```python
from build123d import *

# Parameters (mm, degrees)
SALIENTE_EXTRUIR1_DEPTH = 8.98
CROQUIS2_R              = 7
SALIENTE_EXTRUIR3_DEPTH = 110
CHAFL_N4_SIZE           = 1


with BuildPart() as part:
    # Croquis1 → Saliente-Extruir1 (new body)
    with BuildSketch(Plane(origin=(0, 0, 0), x_dir=(1, 0, 0), z_dir=(0, 1, 0))):
        Polygon((11, 0), (5.5, 9.526279442), (-5.5, 9.526279442), (-11, 0), (-5.5, -9.526279442), (5.5, -9.526279442), align=None)
    extrude(amount=SALIENTE_EXTRUIR1_DEPTH)

    # Croquis2 → Saliente-Extruir3 (add)
    with BuildSketch(Plane(origin=(0, 8.98, 0), x_dir=(1, 0, 0), z_dir=(0, 1, 0))):
        with Locations(Location((0, 0, 0), (0, 0, 270))):
            Circle(CROQUIS2_R)
    extrude(amount=SALIENTE_EXTRUIR3_DEPTH)

    # Chaflán4
    chafl_n4_edges = [part.edges().sort_by_distance(p)[0] for p in [
        (0, 118.98, -7),
    ]]
    chamfer(chafl_n4_edges, length=CHAFL_N4_SIZE)


solid = part.part
```
Design review of the part built by this model. Coordinates are the model's own, in mm. A direction names the side the tool comes from. Round coordinates to 2 decimals unless told otherwise and drop trailing zeros. Write each loop counter-clockwise with the first axis right and the second up, starting at its lowest first coordinate (ties: lowest second). Pieces come first, ordered by that corner, then holes.
Item 1: For probe 1 along Y at (x, z) = (1.25, 7.5); probe 2 along X at (y, z) = (19.5, 0.5); probe 3 along X at (y, z) = (76, -5.5), list the stretches that pass through material, from the lowest coordinate up.
Item 2: Clearance check with flat-ended pins moving along their axes: pin 1 Ø2 at (y, z) = (92.5, -2.5) entering from +X; pin 2 Ø8 at (x, y) = (0.5, 103) entering from -Z; pin 3 Ø10 at (x, y) = (-8, 52) entering from +Z; pin 4 Ø1.5 at (x, y) = (-8.5, 31) entering from +Z. State where each tip first meets the part, or that it passes through.
Item 3: We need section B-B on y = 22.5. Write out the cut boundary in (x, z).
Item 4: For faces 1 (the flat face through (-8.288, 4.427, 4.696)), 2 (the cylindrical face through (-6.834, 62.717, -1.517)), list the 3-axis set-ups (+Z, -Z, +X, -X, +Y, -Y) from which the entire face can be reached by the end or side of a thin tool; tool diameter is ignored.
Item 5: We need section A-A on x = 0. Write out the cut boundary in (y, z).
Returned:
1. probe 1: y = 0 to 8.98
1. probe 2: x = -6.98 to 6.98
1. probe 3: x = -4.33 to 4.33
2. pin 1: stops at x = 6.84
2. pin 2: stops at z = -7
2. pin 3: stops at z = 6.32
2. pin 4: passes through
3. outline: circle Ø14 at (0, 0)
4. face 1: +Z, -X, +Y, -Y
4. face 2: +Y
5. outline: (0, -9.53) - (8.98, -9.53) - (8.98, -7) - (117.98, -7) - (118.98, -6) - (118.98, 6) - (117.98, 7) - (8.98, 7) - (8.98, 9.53) - (0, 9.53) - close
